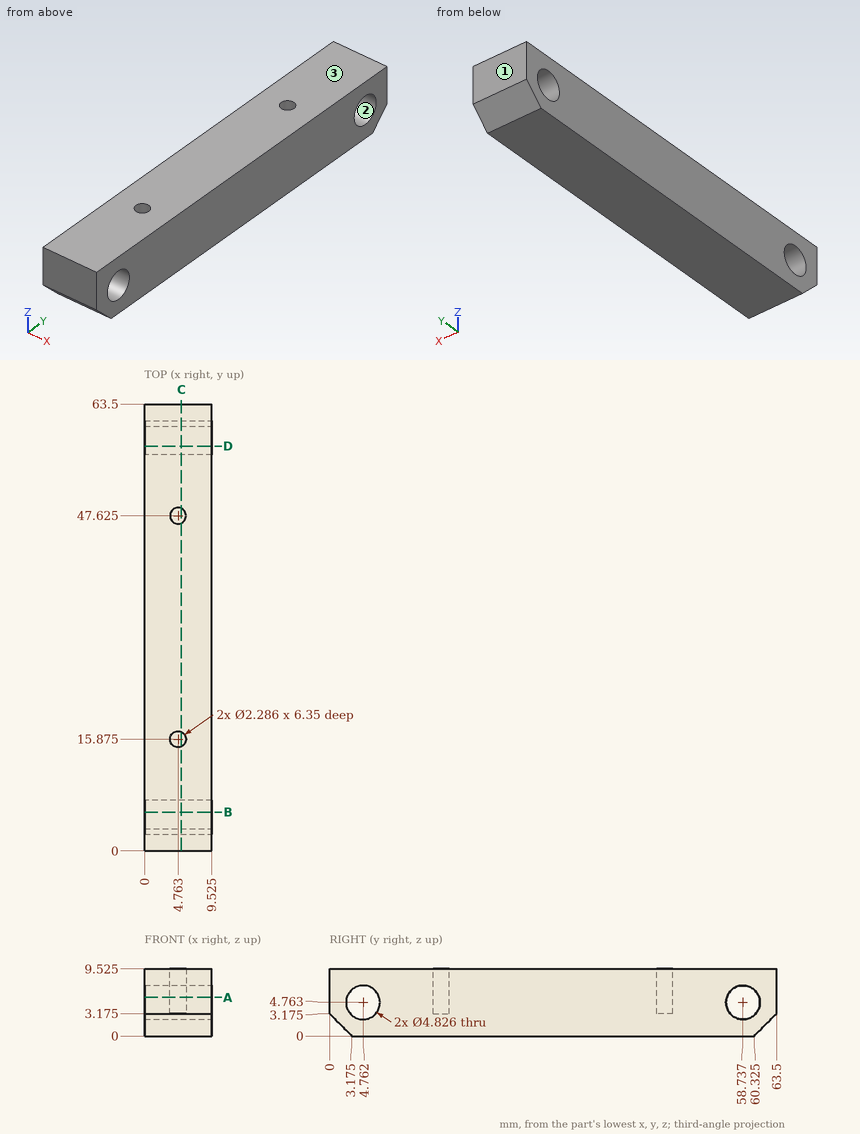
Input: dimensioned drawing with shaded views. Units: mm. Origin: part minimum x, y, z. Give positions to 0.01 mm unless a question says otherwise; leave off trailing zeros. Write each loop counter-clockwise with the first axis right and the second up, starting at its lowest first coordinate (ties: lowest second). Pieces come first, ordered by that corner, then holes.
Q1. Material intervals for probe 1 along Y at (x, z) = (8.5, 5) (1 decimal); probe 2 along Y at (x, z) = (1.5, 3) (1 decimal); probe 3 along Z at (x, y) = (8.75, 4) (1 decimal), sorted ascending.
Q2. Section D-D, the plane y = 57.5. Output: boundary loops of the cut face in (x, z) (1 decimal).
Q3. Section B-B, the plane y = 5.5. Output: boundary loops of the cut face in (x, z) (1 decimal).
Q4. Section A-A, the plane z = 5.5. Output: boundary loops of the cut face in (x, y) (1 decimal).
Q5. Section C-C, the plane x = 5.25. Output: boundary loops of the cut face in (y, z) (1 decimal), plus the area to 3 significant figures.
Q6. First-contact query: P1, Ø4, axis at y = 58.74, z = 4.76, coming from the +X side. Flat tip, straight axial feed; report the tip coordinate or a pass-through.
Q7. Pull-direction query (Y, two-part tool) for the marked faces 1, 2 and 3; classes: pulls with the +Y half, pulls with the -Y half, needs draft (parallel to the pull), parting line crosses it, or undercut.
Filled in:
1. probe 1: y = 0 to 2.4, 7.2 to 56.3, 61.1 to 63.5
1. probe 2: y = 0.2 to 3.1, 6.4 to 57.1, 60.4 to 63.3
1. probe 3: z = 0 to 2.5, 7.1 to 9.5
2. outline: (0, 0) - (9.5, 0) - (9.5, 2.7) - (0, 2.7) - close; (0, 6.8) - (9.5, 6.8) - (9.5, 9.5) - (0, 9.5) - close
3. outline: (0, 0) - (9.5, 0) - (9.5, 2.5) - (0, 2.5) - close; (0, 7.1) - (9.5, 7.1) - (9.5, 9.5) - (0, 9.5) - close
4. outline: (0, 0) - (9.5, 0) - (9.5, 2.5) - (0, 2.5) - close; (0, 7.1) - (9.5, 7.1) - (9.5, 56.4) - (0, 56.4) - close; (0, 61) - (9.5, 61) - (9.5, 63.5) - (0, 63.5) - close; hole circle Ø2.3 at (4.8, 15.9); hole circle Ø2.3 at (4.8, 47.6)
5. outline: (0, 3.2) - (3.2, 0) - (60.3, 0) - (63.5, 3.2) - (63.5, 9.5) - (48.7, 9.5) - (48.7, 3.2) - (46.6, 3.2) - (46.6, 9.5) - (16.9, 9.5) - (16.9, 3.2) - (14.8, 3.2) - (14.8, 9.5) - (0, 9.5) - close; hole circle Ø4.8 at (4.8, 4.8); hole circle Ø4.8 at (58.7, 4.8)
5. area: 532 mm2
6. P1: passes through
7. face 1: pulls with the +Y half
7. face 2: undercut
7. face 3: needs draft
